For this review, take the finished solid that the model builds, in its own axes (mm). A direction names the side the tool comes from. Give positions to 0.01 mm unless a question says otherwise; leave off trailing zeros. Order: outer loops, then holes, each group sorted by start corner. A loop starts at its lowest first (then second) coordinate and runs counter-clockwise, first axis right, second up. Notation, with made-up numbers: (54.5, -37) - (82.5, -37) arc R25 ccw to (82.5, -2) - close; hole circle Ø6 at (80.5, 84.5). An arc over 180 degrees is marked (long way). One line per item, written item: value.
```python
from build123d import *

# Parameters (mm, degrees)
SKETCH011_W     = 189
SKETCH011_H     = 96
SKETCH011_W_2   = 112
SKETCH011_H_2   = 56
PAD010_DEPTH    = 2
SKETCH012_W     = 189
SKETCH012_H     = 96
PAD011_DEPTH    = 9.5
SKETCH013_R     = 1.7
POCKET_DEPTH    = 9
SKETCH014_W     = 6
SKETCH014_H     = 2.8
POCKET001_DEPTH = 12
SKETCH015_W     = 6
SKETCH015_H     = 2.8
POCKET002_DEPTH = 12
SKETCH016_W     = 18
SKETCH016_H     = 10
POCKET003_DEPTH = 11.501
SKETCH017_R     = 2.55
SKETCH017_R_2   = 2.6
POCKET004_DEPTH = 11.501
FILLET_R        = 2.5
FILLET005_R     = 5
FILLET006_R     = 1
POCKET005_DEPTH = 3.5
FILLET007_R     = 3


with BuildPart() as part:
    # Sketch011 → Pad010 (new body)
    with BuildSketch(Plane.XY):
        with Locations((0, 5)):
            Rectangle(SKETCH011_W, SKETCH011_H)
        Rectangle(SKETCH011_W_2, SKETCH011_H_2, mode=Mode.SUBTRACT)
    extrude(amount=PAD010_DEPTH)

    # Sketch012 (on Face9 of Pad010) → Pad011 (join)
    with BuildSketch(Plane(origin=(0, 0, 0), x_dir=(1, 0, 0), z_dir=(0, 0, -1))):
        with Locations((0, -5)):
            Rectangle(SKETCH012_W, SKETCH012_H)
        Polygon((-71, 41), (76, 41), (76, -33), (-71, -33), (-71, -7), (-82.050253, -7), (-87, -11.949747), (-87, -34), (-92, -34), (-92, 12), (-71, 12), align=None, mode=Mode.SUBTRACT)
    extrude(amount=PAD011_DEPTH)

    # Sketch013 (on Face9 of Pad011) → Pocket (cut)
    with BuildSketch(Plane(origin=(0, 0, -9.5), x_dir=(1, 0, 0), z_dir=(0, 0, -1))):
        with Locations((-86.5, 37)):
            Circle(SKETCH013_R)
        with Locations((-86.5, -47)):
            Circle(SKETCH013_R)
        with Locations((86.5, 37)):
            Circle(SKETCH013_R)
        with Locations((86.5, -47)):
            Circle(SKETCH013_R)
    extrude(amount=-POCKET_DEPTH, mode=Mode.SUBTRACT)

    # Sketch014 (on Face7 of Pocket) → Pocket001 (cut)
    with BuildSketch(Plane(origin=(-94.5, 0, 0), x_dir=(0, -1, 0), z_dir=(-1, 0, 0))):
        with Locations((36.9, -4.6)):
            Rectangle(SKETCH014_W, SKETCH014_H)
        with Locations((-46.9, -4.6)):
            Rectangle(SKETCH014_W, SKETCH014_H)
    extrude(amount=-POCKET001_DEPTH, mode=Mode.SUBTRACT)

    # Sketch015 (on Face8 of Pocket001) → Pocket002 (cut)
    with BuildSketch(Plane.YZ.offset(94.5)):
        with Locations((-36.9, -4.6)):
            Rectangle(SKETCH015_W, SKETCH015_H)
        with Locations((46.9, -4.6)):
            Rectangle(SKETCH015_W, SKETCH015_H)
    extrude(amount=-POCKET002_DEPTH, mode=Mode.SUBTRACT)

    # Sketch016 (on Face9 of Pocket002) → Pocket003 (cut, through all)
    with BuildSketch(Plane(origin=(0, 0, -9.5), x_dir=(1, 0, 0), z_dir=(0, 0, -1))):
        with Locations((-9, -33)):
            Rectangle(SKETCH016_W, SKETCH016_H)
    extrude(amount=-POCKET003_DEPTH, mode=Mode.SUBTRACT)

    # Sketch017 (on Face9 of Pocket003) → Pocket004 (cut, through all)
    with BuildSketch(Plane(origin=(0, 0, -9.5), x_dir=(1, 0, 0), z_dir=(0, 0, -1))):
        with Locations((-58.5, -45.5)):
            Circle(SKETCH017_R)
        with Locations((-45.5, -45.5)):
            Circle(SKETCH017_R)
        with Locations((-32.5, -45.5)):
            Circle(SKETCH017_R)
        with Locations((-19.5, -45.5)):
            Circle(SKETCH017_R)
        with Locations((-6.5, -45.5)):
            Circle(SKETCH017_R)
        with Locations((6.5, -45.5)):
            Circle(SKETCH017_R)
        with Locations((19.5, -45.5)):
            Circle(SKETCH017_R)
        with Locations((32.5, -45.5)):
            Circle(SKETCH017_R)
        with Locations((45.5, -45.5)):
            Circle(SKETCH017_R)
        with Locations((58.5, -45.5)):
            Circle(SKETCH017_R)
        with Locations((-80.7, -12)):
            Circle(SKETCH017_R_2)
        with Locations((-80.7, -21)):
            Circle(SKETCH017_R_2)
        with Locations((-80.7, -30)):
            Circle(SKETCH017_R_2)
        with Locations((80.7, -12)):
            Circle(SKETCH017_R_2)
        with Locations((80.7, -21)):
            Circle(SKETCH017_R_2)
        with Locations((80.7, -30)):
            Circle(SKETCH017_R_2)
    extrude(amount=-POCKET004_DEPTH, mode=Mode.SUBTRACT)

    # Fillet
    fillet_edges = [part.edges().sort_by_distance(p)[0] for p in [
        (-94.5, 53, -4.75),
        (-94.5, -43, -4.75),
        (94.5, -43, -4.75),
        (94.5, 53, -4.75),
    ]]
    fillet(fillet_edges, radius=FILLET_R)

    # Fillet005
    fillet005_edges = [part.edges().sort_by_distance(p)[0] for p in [
        (76, -41, -4.75),
    ]]
    fillet(fillet005_edges, radius=FILLET005_R)

    # Fillet006
    fillet006_edges = [part.edges().sort_by_distance(p)[0] for p in [
        (83.3, 30, -3.75),
        (-78.1, 12, -3.75),
        (35.05, 45.5, -3.75),
        (83.3, 21, -3.75),
        (48.05, 45.5, -3.75),
        (-78.1, 30, -3.75),
        (-78.1, 21, -3.75),
        (-71, -41, -4.75),
    ]]
    fillet(fillet006_edges, radius=FILLET006_R)

    # Sketch018 (on Face1 of Fillet006) → Pocket005 (cut)
    with BuildSketch(Plane(origin=(0, 0, -9.5), x_dir=(1, 0, 0), z_dir=(0, 0, -1))):
        Polygon((-87, -5), (-87, -35.5), (-72.5, -50), (72.5, -50), (87, -35.5), (87, -5), (70, -5), (70, -39), (-70, -39), (-70, -5), align=None)
    extrude(amount=-POCKET005_DEPTH, mode=Mode.SUBTRACT)

    # Fillet007
    fillet007_edges = [part.edges().sort_by_distance(p)[0] for p in [
        (-18, 38, -3.75),
        (0, 38, -3.75),
    ]]
    fillet(fillet007_edges, radius=FILLET007_R)


with BuildPart() as part_1:
    # Body007 placement: moved
    add(part.part.moved(Location((0, 82, 15))))


solid = part_1.part
```
(1) Take a section at A-A (x = -39). Write out the cut boundary in (y, z).
Answers below:
outline: (39, 5.5) - (41, 5.5) - (41, 15) - (54, 15) - (54, 17) - (39, 17) - close; (110, 15) - (115, 15) - (115, 5.5) - (121, 5.5) - (121, 9) - (132, 9) - (132, 5.5) - (135, 5.5) - (135, 17) - (110, 17) - close
(2) Take a section at B-B (y = 83). Write out the cut boundary in (x, z).
Answers below:
outline: (-94.5, 5.5) - (-92, 5.5) - (-92, 15) - (-56, 15) - (-56, 17) - (-94.5, 17) - close; (56, 15) - (76, 15) - (76, 5.5) - (94.5, 5.5) - (94.5, 17) - (56, 17) - close
(3) Wall thickness on line 1 (Y direction, x = -58.5, z = 13); line 2 (Y direction, x = 81, z = 12.5); line 3 (X direction, y = 106, z = 12.5): over which ranges is each line inside the solid? List them lowest first. Write a range as from..to.
Answers below:
line 1: y = 39..41, 115..124.95, 130.05..135
line 2: y = 39..91.42, 96.58..100.42, 105.58..109.42, 114.58..135
line 3: x = -94.5..-92, -87..-71, 76..94.5
(4) Draft analysis for pull direction Y (two halves, no side actions). For faces 4 (the face through (-1, 39, 11)), 5 (the face through (-47.4, 125.8, 12.9)), 6 (the face through (-1, 135, 11)), state which applies: pulls with the +Y half, pulls with the -Y half, needs draft (parallel to the pull), parting line crosses it, or undercut.
Answers below:
face 4: pulls with the -Y half
face 5: undercut
face 6: pulls with the +Y half
(5) Machinability: for faces 1 (the face through (84.8, 128.93, 13.13)), 2 (the face through (89, 129, 11.8)), 3 (the face through (-89, 129, 9)), which of the approach directions +Z, -Z, +X, -X, +Y, -Y give a long, thin tool a straight path to every point of the face, cutting with its end or side? Answer none if there is none.
Answers below:
face 1: -Z
face 2: +X
face 3: -X
(6) For P1, Ø5.5, axis at x = -86.5, y = 129, coming from the -Z side; P2, Ø8.5, axis at x = -80.7, y = 112, coming from the -Z side, all flat-tipped, find the tip position at first contact; note any pin that passes through.
Answers below:
P1: stops at z = 5.5
P2: stops at z = 9
(7) Take a section at D-D (y = 103). Write out the cut boundary in (x, z), then the cut area to 3 significant figures.
Answers below:
outline: (-94.5, 5.5) - (-92, 5.5) - (-92, 15) - (-87, 15) - (-87, 9) - (-83.3, 9) - (-83.3, 17) - (-94.5, 17) - close; (-78.1, 9) - (-71, 9) - (-71, 15) - (-56, 15) - (-56, 17) - (-78.1, 17) - close; (56, 15) - (76, 15) - (76, 9) - (78.1, 9) - (78.1, 17) - (56, 17) - close; (83.3, 9) - (87, 9) - (87, 5.5) - (94.5, 5.5) - (94.5, 17) - (83.3, 17) - close
area: 328 mm^2
(8) Take a section at C-C (x = -6.5). Write out the cut boundary in (y, z).
Answers below:
outline: (39, 5.5) - (41, 5.5) - (41, 15) - (54, 15) - (54, 17) - (39, 17) - close; (120, 5.5) - (121, 5.5) - (121, 9) - (124.95, 9) - (124.95, 17) - (120, 17) - close; (130.05, 9) - (132, 9) - (132, 5.5) - (135, 5.5) - (135, 17) - (130.05, 17) - close
